Geometry check sheet. Reference: the model listing, model coordinates, mm. A direction names the side the tool comes from. Round coordinates to 2 decimals unless told otherwise and drop trailing zeros. Order: outer loops, then holes, each group sorted by start corner. A loop starts at its lowest first (then second) coordinate and runs counter-clockwise, first axis right, second up. Notation, with made-up numbers: (-11.5, 76) - (8.5, 76) arc R19 ccw to (8.5, 100) - close; hole circle Ø1 at (52.25, 63). An arc over 180 degrees is marked (long way). Return JSON: item names as keys, results as strings. Group by question number.
Q1. Gauge pin test, flat ends, axial feed: pin 1 Ø2 at (x, y) = (-203, 17) entering from -Z; pin 2 Ø6.5 at (y, z) = (-164, 27) entering from -X; pin 3 Ø3 at (x, z) = (81, 47) entering from -Y. Record the tip position at first contact, or that the pin passes through.
Q2. Draft check along Y on faces 1 (the flat face through (199, -160, 40)), 2 (the flat face through (-2.81, -164.81, 26.92)), 3 (the flat face through (-2.8, -162.9, 25.9)). Enter one of: pulls with the +Y half, pulls with the -Y half, needs draft (parallel to the pull), parting line crosses it, or undercut.
Q3. Sectioned sample at A-A, the plane z = 32.5. Record the cut outline in (x, y).
Q4. Material ranges on line 1 along X through (y, z) = (122, 40.5); line 2 along X through (y, z) = (107, 0); line 3 along Y through (x, z) = (-126, 36), recorded low to high.
Q5. Tool access check on faces 4 (the flat face through (-199, 160, 40)), 5 (the flat face through (-199.9, -2.3, 25.9)), 6 (the flat face through (-199, -160, 40)), 7 (the flat face through (199, 160, 40)). Record the directions out of +Z, -Z, +X, -X, +Y, -Y that give a thin tool (end or side, any length) a straight path to the whole face; none if there is none.
Solid Edge part; units mm, degrees
sketch "Sketch1" plane through (0, 0, 0) normal (0, 0, 1) x (1, 0, 0)
  line L0 (-204.5, -167.5) -> (204.5, -167.5)
  line L1 (204.5, -167.5) -> (204.5, 167.5)
  line L2 (204.5, 167.5) -> (-204.5, 167.5)
  line L3 (-204.5, 167.5) -> (-204.5, -167.5)
  dimension "D1" = 204.5
  dimension "D2" = 204.5
extrude "Protrusion1" add sketch "Sketch1" along normal blind 60
sketch "Sketch2" plane through (0, -167.5, 30) normal (0, -1, 0) x (1, 0, 0)
  line L0 (-204.5, -30) -> (-198.5, 30)
  line L1 (-198.5, 30) -> (-204.5, 30)
  line L2 (-204.5, 30) -> (-204.5, -30)
  line L3 (198.5, 30) -> (204.5, -30)
  line L4 (204.5, -30) -> (204.5, 30)
  line L5 (204.5, 30) -> (198.5, 30)
  dimension "D1" = 198.5
  dimension "D2" = 204.5
extrude "Cutout1" cut sketch "Sketch2" against normal up to next
sketch "Sketch3" plane through (-210, 0, 0) normal (-1, 0, 0) x (0, -1, 0)
  line L0 (-167.5, 0) -> (-161.5, 60)
  line L1 (-161.5, 60) -> (-167.5, 60)
  line L2 (-167.5, 60) -> (-167.5, 0)
  line L3 (167.5, 0) -> (161.5, 60)
  line L4 (161.5, 60) -> (167.5, 60)
  line L5 (167.5, 60) -> (167.5, 0)
  dimension "D1" = 161.5
  dimension "D2" = 161.5
extrude "Cutout_2" cut sketch "Sketch3" against normal up to next
shell "Thin_Wall" thickness 2 removed faces 1 at (-140.4233, -108.3167, 0)
sketch "Sketch4" plane through (0, 0, 0) normal (0, 0, -1) x (-1, 0, 0)
  line L0 (204.5, 165.49) -> (204.5, -167.5)
  line L1 (204.5, -167.5) -> (-204.5, -167.5)
  line L2 (-204.5, -167.5) -> (-204.5, 165.49)
  line L3 (-202.49, 165.49) -> (-204.5, 165.49)
  line L4 (-202.49, -165.49) -> (-202.49, 165.49)
  line L5 (202.49, -165.49) -> (-202.49, -165.49)
  line L6 (202.49, 165.49) -> (202.49, -165.49)
  line L7 (202.49, 165.49) -> (204.5, 165.49)
extrude "Attachment" add sketch "Sketch4" along normal blind 1
sketch "Sketch5" plane through (0, 0, -1) normal (0, 0, -1) x (0, 1, 0)
  line L0 (-167.5, 204.5) -> (-151.5, 204.5)
  line L1 (-151.5, 204.5) -> (-151.5, 188.5)
  line L2 (-151.5, 188.5) -> (-167.5, 188.5)
  line L3 (-167.5, 188.5) -> (-167.5, 204.5)
  line L4 (167.5, 204.5) -> (151.5, 204.5)
  line L5 (151.5, 204.5) -> (151.5, 188.5)
  line L6 (151.5, 188.5) -> (167.5, 188.5)
  line L7 (167.5, 188.5) -> (167.5, 204.5)
  line L8 (167.5, -204.5) -> (151.5, -204.5)
  line L9 (151.5, -204.5) -> (151.5, -188.5)
  line L10 (151.5, -188.5) -> (167.5, -188.5)
  line L11 (167.5, -188.5) -> (167.5, -204.5)
  line L12 (-167.5, -204.5) -> (-151.5, -204.5)
  line L13 (-151.5, -204.5) -> (-151.5, -188.5)
  line L14 (-151.5, -188.5) -> (-167.5, -188.5)
  line L15 (-167.5, -188.5) -> (-167.5, -204.5)
  dimension "D1" = 151.5
  dimension "D2" = 151.5
extrude "Cutout___Pillars" cut sketch "Sketch5" against normal blind 41
fillet "Round___Top" radius 6 8 edges at (0, -161.5, 60) (198.5, 0, 60) (0, 161.5, 60) (-198.5, 0, 60) (0, -159.69, 58) (196.69, 0, 58) (0, 159.69, 58) (-196.69, 0, 58)
sketch "Sketch6" plane through (-188.5, 0, 0) normal (1, 0, 0) x (0, 1, 0)
  line L0 (165.49, 0) -> (166.49, -10)
  line L1 (166.49, -10) -> (168.5, -10)
  line L2 (168.5, -10) -> (167.5, 0)
  line L3 (167.5, 0) -> (165.49, 0)
extrude "Front" add sketch "Sketch6" along normal blind 377
properties material "Glass, general industrial"
Reply:
{
 "1": {"pin 1": "z = -1", "pin 2": "x = -188.5", "pin 3": "y = -162.95"},
 "2": {"face 1": "needs draft", "face 2": "pulls with the -Y half", "face 3": "undercut"},
 "3": {"outline": "(-201.25, -151.5) - (-199.24, -151.5) - (-199.24, 151.5) - (-201.25, 151.5) - close; (-188.5, -164.25) - (188.5, -164.25) - (188.5, -162.24) - (-188.5, -162.24) - close; (-188.5, 162.24) - (188.5, 162.24) - (188.5, 164.25) - (-188.5, 164.25) - close; (199.24, -151.5) - (201.25, -151.5) - (201.25, 151.5) - (199.24, 151.5) - close"},
 "4": {"line 1": "-200.45 to -198.44, 198.44 to 200.45", "line 2": "-204.5 to -202.49, 202.49 to 204.5", "line 3": "-163.9 to -161.89, 161.89 to 163.9"},
 "5": {"face 4": "-Z, -X, +Y", "face 5": "-Z", "face 6": "-Z, -X, -Y", "face 7": "-Z, +X, +Y"}
}
